Geometry: see drawing. Coordinates: mm, zero at the bounding-box minimum. A direction names the side the tool comes from. Give positions to 0.01 mm unless a question says otherwise; leave off trailing zeros. Loops run counter-clockwise (first coordinate to the right, second up) from the corner with the lowest first, then second, coordinate; pieces in that order, holes last. Notation, with made-up numbers: M 48,66 L 87,66 A20 ccw 87,96 Z; hole C 32,88.5 d8. An arc over 180 degrees is marked long. Use a Markdown table: item, result. Add a question column.
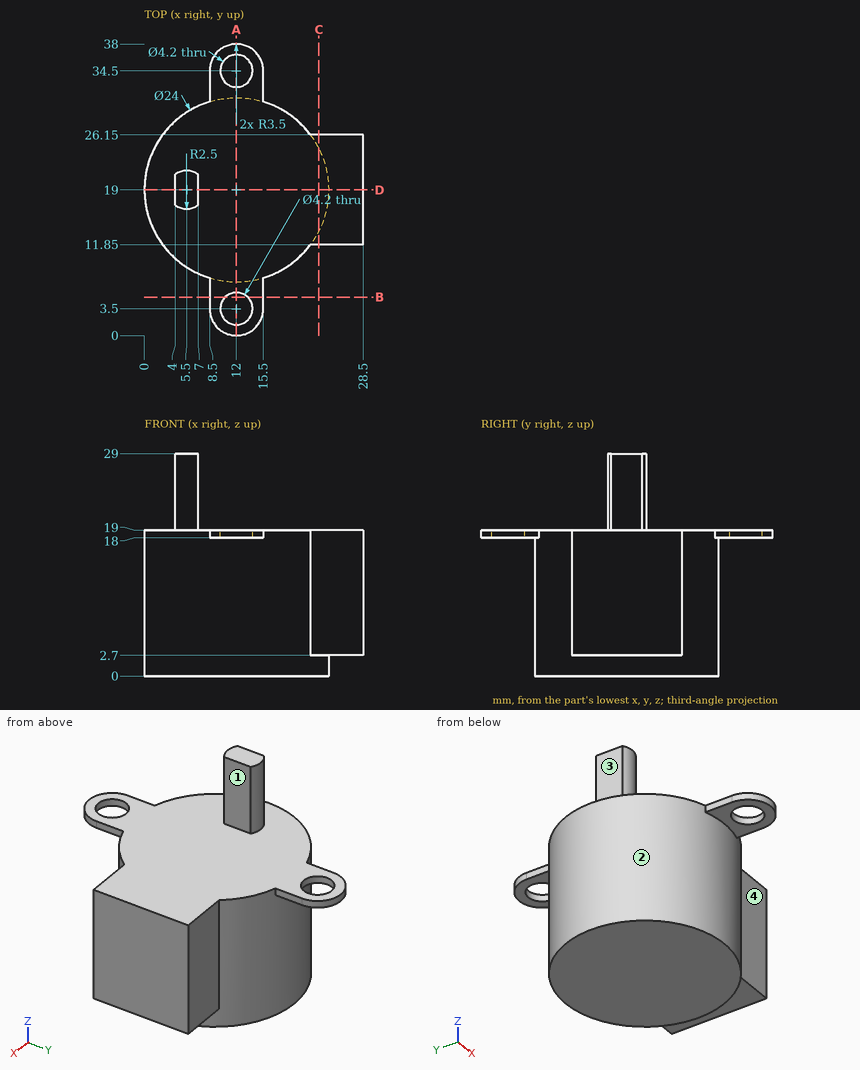
1) Ray query, line 1 (X direction, y = 34.5, z = 18.5); line 2 (Y direction, x = 11.5, z = 8.25); line 3 (Z direction, x = 14.5, y = 4). Return the intervals inside material, ascending. Write a range as [from, to].
2) Section query D-D, the plane y = 19. Return the cut outline in (x, z).
3) Section query A-A, the plane x = 12. Return the cut outline in (y, z), and give its area (3 significant figures).
4) Section query B-B, the plane y = 5. Return the cut outline in (x, z).
5) Contact query for flat-ended pins moving along their axis: P1, Ø4, axis at x = 17.5, z = 11, coming from the -Y side; P2, Ø0.5, axis at y = 6.5, z = 18.5, coming from the -X side; P3, Ø6, axis at x = 21, z = 8.5, coming from the +Y side; P4, Ø3.5, axis at x = 12, y = 34.5, coming from the -Z side. Output: stop coordinate, or through.
6) Section query C-C, the plane x = 22.75. Return the cut outline in (y, z).
7) Reachability of the marked faces 1, 2, 3 and 4 from +Z, -Z, +X, -X, +Y, -Y: full face, straight path, thin tool, end or side. Return the list, or none.
Entries:
| question | item | result |
|---|---|---|
| 1 | line 1 | x = [8.5, 9.9], [14.1, 15.5] |
| 1 | line 2 | y = [7.01, 30.99] |
| 1 | line 3 | z = [18, 19] |
| 2 | outline | M 0,0 L 24,0 L 24,2.7 L 28.5,2.7 L 28.5,19 L 7,19 L 7,29 L 4,29 L 4,19 L 0,19 Z |
| 3 | outline | M 0,18 L 1.4,18 L 1.4,19 L 0,19 Z; M 5.6,18 L 7,18 L 7,0 L 31,0 L 31,18 L 32.4,18 L 32.4,19 L 5.6,19 Z; M 36.6,18 L 38,18 L 38,19 L 36.6,19 Z |
| 3 | area | 462 mm² |
| 4 | outline | M 8.5,18 L 10.53,18 L 10.53,19 L 8.5,19 Z; M 13.47,18 L 15.5,18 L 15.5,19 L 13.47,19 Z |
| 5 | P1 | stops at y = 7.52 |
| 5 | P2 | stops at x = 8.5 |
| 5 | P3 | stops at y = 29.39 |
| 5 | P4 | passes through |
| 6 | outline | M 11.85,2.7 L 13.67,2.7 L 13.67,0 L 24.33,0 L 24.33,2.7 L 26.15,2.7 L 26.15,19 L 11.85,19 Z |
| 7 | face 1 | +Z, +X, +Y, -Y |
| 7 | face 2 | -Z |
| 7 | face 3 | +Z, -X, +Y, -Y |
| 7 | face 4 | +Z, -Z, +X, -Y |
